Design review of the part shown in the three views and the two pictorial views. Dimensions are in mm from the part's minimum x, y and z. A direction names the side the tool comes from. Give positions to 0.01 mm unless a question says otherwise; leave off trailing zeros. Order: outer loops, then holes, each group sorted by start corner. A loop starts at its lowest first (then second) coordinate and runs counter-clockwise, first axis right, second up.
Item 1: Consider section D-D (x = 1.5). Give the boundary of the cut face in (y, z).
Item 2: The part is to be moulded in two halves that separate along Z. For the marked faces 6, 7 and 8, say which applies: released by +Z, released by -Z, zero draft, split by the parting line, or undercut.
Item 3: Consider section A-A (y = 0.5). Give the boundary of the cut face in (x, z).
Item 4: For P1, Ø3, axis at x = 3, y = 5, coming from the -Z side; P2, Ø1.9, axis at x = 4, z = 2.5, coming from the +Y side; P3, Ø1.5, axis at x = 4.5, y = 5, coming from the +Z side; P4, Ø2.5, axis at x = 2.5, z = 3.5, coming from the +Y side, all flat-tipped, find the tip position at first contact; note any pin that passes through.
Item 5: For probe 1 along Z at (x, y) = (4, 1.25); probe 2 along X at (y, z) = (0.5, 19.5); probe 3 along Z at (x, y) = (5.75, 0.75), list the stretches that pass through material, from the lowest coordinate up.
Item 6: Consider section B-B (x = 4). Give the boundary of the cut face in (y, z), plus the area to 3 significant figures.
Item 7: Consider section C-C (z = 19.5). Give the boundary of the cut face in (x, y), plus the area to 3 significant figures.
Item 8: Machinability: for the marked faces 1, 2, 3, 4 and 5, which of the approach directions +Z, -Z, +X, -X, +Y, -Y give a long, thin tool a straight path to every point of the face, cutting with its end or side? Answer none if there is none.
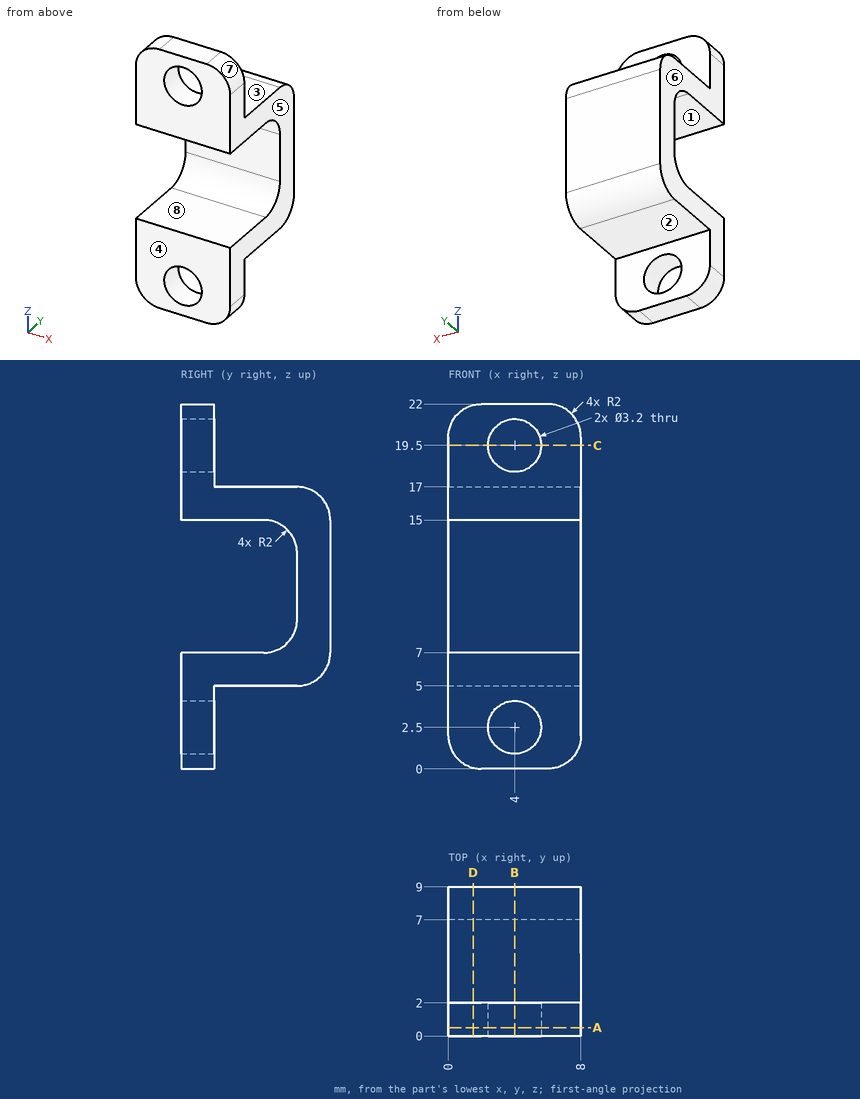
Resolved:
1. outline: (0, 0.06) - (2, 0.06) - (2, 5) - (7, 5) arc R2 ccw to (9, 7) - (9, 15) arc R2 ccw to (7, 17) - (2, 17) - (2, 21.94) - (0, 21.94) - (0, 15) - (5, 15) arc R2 cw to (7, 13) - (7, 9) arc R2 cw to (5, 7) - (0, 7) - close
2. face 6: zero draft
2. face 7: released by +Z
2. face 8: undercut
3. outline: (0, 2) arc R2 ccw to (2, 0) - (6, 0) arc R2 ccw to (8, 2) - (8, 7) - (0, 7) - close; (0, 15) - (8, 15) - (8, 20) arc R2 ccw to (6, 22) - (2, 22) arc R2 ccw to (0, 20) - close; hole circle Ø3.2 at (4, 2.5); hole circle Ø3.2 at (4, 19.5)
4. P1: stops at z = 5
4. P2: passes through
4. P3: stops at z = 17
4. P4: stops at y = 2
5. probe 1: z = 0 to 0.9, 4.1 to 7, 15 to 17.9, 21.1 to 22
5. probe 2: x = 0 to 2.4, 5.6 to 8
5. probe 3: z = 0 to 7, 15 to 22
6. outline: (0, 0) - (2, 0) - (2, 0.9) - (0, 0.9) - close; (0, 4.1) - (2, 4.1) - (2, 5) - (7, 5) arc R2 ccw to (9, 7) - (9, 15) arc R2 ccw to (7, 17) - (2, 17) - (2, 17.9) - (0, 17.9) - (0, 15) - (5, 15) arc R2 cw to (7, 13) - (7, 9) arc R2 cw to (5, 7) - (0, 7) - close; (0, 21.1) - (2, 21.1) - (2, 22) - (0, 22) - close
6. area: 59.2 mm2
7. outline: (0, 0) - (2.4, 0) - (2.4, 2) - (0, 2) - close; (5.6, 0) - (8, 0) - (8, 2) - (5.6, 2) - close
7. area: 9.60 mm2
8. face 1: +X, -X, -Y
8. face 2: -Z, +X, -X, +Y
8. face 3: +Z, +X, -X, +Y
8. face 4: +Z, -Z, +X, -X, -Y
8. face 5: +Z, -Z, +X, +Y, -Y
